from build123d import *

# Parameters (mm, degrees)
F0_W      = 50
F0_H      = 50
F1_DEPTH  = 3
F2_W      = 3
F2_H      = 3
F2_H_2    = 47
F3_DEPTH  = 50
F4_W      = 3
F4_H      = 50
F5_DEPTH  = 47
F6_DEPTH  = 3
F7_W      = 3.2
F7_H      = 3.2
F8_DEPTH  = 50
F9_W      = 40.8
F9_H      = 3
F10_DEPTH = 40.8
F11_R     = 2


with BuildPart() as f1:
    # F0 (on Top) → F1 (new body)
    with BuildSketch(Plane.XY):
        Rectangle(F0_W, F0_H)
    extrude(amount=F1_DEPTH)

    # F2 (on face) → F3 (join, through all)
    with BuildSketch(Plane(origin=(-25, 0, 0), x_dir=(0, -1, 0), z_dir=(-1, 0, 0))):
        with Locations((-23.5, 1.5)):
            Rectangle(F2_W, F2_H)
        with Locations((-17.3, 1.5)):
            Rectangle(F2_W, F2_H)
        with Locations((-17.3, -23.5)):
            Rectangle(F2_W, F2_H_2)
        with Locations((-23.5, -23.5)):
            Rectangle(F2_W, F2_H_2)
    extrude(amount=-F3_DEPTH)

    # F4 (on face) → F5 (join, through all)
    with BuildSketch(Plane.XZ.offset(25)):
        with Locations((23.5, -22)):
            Rectangle(F4_W, F4_H)
        with Locations((17.3, -22)):
            Rectangle(F4_W, F4_H)
    extrude(amount=-F5_DEPTH)

    # F6 (add, through all): a face of the model
    f6_faces = [f1.faces().sort_by_distance(p)[0] for p in [
        (20.4, 20.4, 0),
    ]]
    extrude(f6_faces, amount=-F6_DEPTH)

    # F7 (on face) → F8 (join, through all)
    with BuildSketch(Plane(origin=(0, 0, -47), x_dir=(1, 0, 0), z_dir=(0, 0, -1))):
        with Locations((20.4, -20.4)):
            Rectangle(F7_W, F7_H)
    extrude(amount=-F8_DEPTH)

    # F9 (on face) → F10 (join, through all)
    with BuildSketch(Plane(origin=(-25, 0, 0), x_dir=(0, -1, 0), z_dir=(-1, 0, 0))):
        with Locations((4.6, -4.7)):
            Rectangle(F9_W, F9_H)
    extrude(amount=-F10_DEPTH)

    # F11
    f11_edges = [f1.edges().sort_by_distance(p)[0] for p in [
        (-25, 0, 3),
        (0, -25, 3),
        (0, 25, 3),
        (25, 0, 3),
        (25, 0, -47),
        (25, -25, -22),
        (25, 25, -22),
        (-25, 25, -22),
        (0, 25, -47),
        (15.8, -25, -26.6),
        (15.8, -4.6, -47),
        (15.8, 15.8, -26.6),
        (15.8, -4.6, -6.2),
        (-25, 15.8, -26.6),
        (-4.6, 15.8, -6.2),
        (-4.6, 15.8, -47),
        (-4.6, -25, -6.2),
        (-25, -4.6, -6.2),
    ]]
    fillet(f11_edges, radius=F11_R)


solid = f1.part
Build history of the part. All positions in model axes, mm. A direction names the side the tool comes from. Give positions to 0.01 mm unless a question says otherwise; leave off trailing zeros. Loops run counter-clockwise (first coordinate to the right, second up) from the corner with the lowest first, then second, coordinate; pieces in that order, holes last. Notation, with made-up numbers: (61.5, 74.25) -> (106.5, 74.25) arc R9 cw to (106.5, 87.25) -> close; hole circle Ø4 at (13, 66). An arc over 180 degrees is marked (long way). Answer in a Markdown table with one row per item.
Item 1: Mould opens along Z. For faces 1 (the cylindrical face through (24.43, -0.32, 2.4)), 2 (the flat face through (25, 0, -22)), 3 (the flat face through (-5, -4, -3.2)), 4 (the flat face through (20, -4, 0)) say: pulls with the +Z half, pulls with the -Z half, needs draft (parallel to the pull), parting line crosses it, or undercut.
Findings below:
| item | result |
|---|---|
| face 1 | pulls with the +Z half |
| face 2 | needs draft |
| face 3 | undercut |
| face 4 | pulls with the -Z half |
Item 2: Slice it at A-A on x = -10. Write the cut outline in (y, z), plus the area to 3 significant figures.
Findings below:
| item | result |
|---|---|
| outline | (-25, -4.2) arc R2 ccw to (-23, -6.2) -> (13.8, -6.2) arc R2 cw to (15.8, -8.2) -> (15.8, -45) arc R2 ccw to (17.8, -47) -> (18.8, -47) -> (18.8, 0) -> (22, 0) -> (22, -47) -> (23, -47) arc R2 ccw to (25, -45) -> (25, 1) arc R2 ccw to (23, 3) -> (-23, 3) arc R2 ccw to (-25, 1) -> (-25, 0) -> (15.8, 0) -> (15.8, -3.2) -> (-25, -3.2) -> close |
| area | 551 mm² |
Item 3: Flat gauge pins, fed straight in: P1, Ø11, axis at y = -11, z = -30, coming from the -X side; P2, Ø1.6, axis at x = -12.5, z = -2, coming from the -Y side; P3, Ø2, axis at x = 14, z = -25, coming from the -Y side. Where does each tip first touch, or does it go through?
Findings below:
| item | result |
|---|---|
| P1 | stops at x = 15.8 |
| P2 | stops at y = 15.8 |
| P3 | stops at y = 15.4 |
Item 4: Probe line 1 along Z through (x, y) = (-11.5, 4); line 2 along X through (y, z) = (4, -40.5). List the from-to ranges inside material, lowest first. Write a range as [from, to].
Findings below:
| item | result |
|---|---|
| line 1 | z = [-6.2, -3.2], [0, 3] |
| line 2 | x = [15.8, 18.8], [22, 25] |
Item 5: Slice it at B-B on z = -19. Write the cut outline in (x, y), plus the area to 3 significant figures.
Findings below:
| item | result |
|---|---|
| outline | (-25, 17.8) arc R2 ccw to (-23, 15.8) -> (13.8, 15.8) arc R2 cw to (15.8, 13.8) -> (15.8, -23) arc R2 ccw to (17.8, -25) -> (18.8, -25) -> (18.8, 15.8) -> (22, 15.8) -> (22, -25) -> (23, -25) arc R2 ccw to (25, -23) -> (25, 23) arc R2 ccw to (23, 25) -> (-23, 25) arc R2 ccw to (-25, 23) -> (-25, 22) -> (15.8, 22) -> (15.8, 18.8) -> (-25, 18.8) -> close |
| area | 571 mm² |
Item 6: Slice it at C-C on x = 19.5. Write the cut outline in (y, z).
Findings below:
| item | result |
|---|---|
| outline | (-25, 0) -> (15.8, 0) -> (15.8, -47) -> (23, -47) arc R2 ccw to (25, -45) -> (25, 1) arc R2 ccw to (23, 3) -> (-23, 3) arc R2 ccw to (-25, 1) -> close |
Item 7: Tool access for faces 5 (the flat face through (20, 15.8, -24)), 6 (the flat face through (-5, 20, 0)), 7 (the flat face through (0, 0, 3)), 8 (the cylindrical face through (16.4, -5.33, -46.43)): list every direction of +Z, -Z, +X, -X, +Y, -Y with a clear straight run to the whole face (end or side of a thin tool).
Findings below:
| item | result |
|---|---|
| face 5 | -Z, -Y |
| face 6 | -Z, -X |
| face 7 | +Z, +X, -X, +Y, -Y |
| face 8 | -Z, -X, -Y |
